Check sheet for the modelled part. Datum: model origin and axes. Units: mm. A direction names the side the tool comes from. Give positions to 0.01 mm unless a question says otherwise; leave off trailing zeros. Order: outer loops, then holes, each group sorted by start corner. A loop starts at its lowest first (then second) coordinate and runs counter-clockwise, first axis right, second up.
```python
from build123d import *

# Parameters (mm, degrees)
SKETCH1_R           = 1.5
BOSS_EXTRUDE1_DEPTH = 1
SKETCH2_R           = 1
BOSS_EXTRUDE2_DEPTH = 2.54


with BuildPart() as part:
    # Sketch1 → Boss-Extrude1 (new body, symmetric)
    with BuildSketch(Plane(origin=(0, 0, 0), x_dir=(1, 0, 0), z_dir=(0, 1, 0))):
        Circle(SKETCH1_R)
    extrude(amount=BOSS_EXTRUDE1_DEPTH, both=True)

    # Sketch2 → Boss-Extrude2 (add)
    with BuildSketch(Plane(origin=(0, 1, 0), x_dir=(1, 0, 0), z_dir=(0, 1, 0))):
        Circle(SKETCH2_R)
    boss_extrude2 = extrude(amount=BOSS_EXTRUDE2_DEPTH)

    # Mirror1: Boss-Extrude2 across plane
    add(boss_extrude2.mirror(Plane.ZX))


solid = part.part
```
(1) Set-up check for faces 1 (the face through (0, 2, 1)), 2 (the face through (0, -2, 1)), 3 (the face through (0, -3.54, 0)): record each of +Z, -Z, +X, -X, +Y, -Y from which the full face is reachable in a straight line by a thin tool's end or side.
Response values:
face 1: +Y
face 2: -Y
face 3: +Z, -Z, +X, -X, -Y
(2) Cross-section at B-B on z = 0. Enter the section's corners in (x, y), then the cut area to 3 significant figures.
Response values:
outline: (-1.5, -1) - (-1, -1) - (-1, -3.54) - (1, -3.54) - (1, -1) - (1.5, -1) - (1.5, 1) - (1, 1) - (1, 3.54) - (-1, 3.54) - (-1, 1) - (-1.5, 1) - close
area: 16.2 mm2
(3) Material ranges on L1, parallel to Y at x = -1, z = -0.85; L2, parallel to Z at x = 0.7, y = 1.5; L3, parallel to X at y = 1.25, z = -0.3, recorded low to high.
Response values:
L1: y = -1 to 1
L2: z = -0.71 to 0.71
L3: x = -0.95 to 0.95
(4) Cross-section at A-A on x = 0. Enter the section's corners in (y, z), then the cut area to 3 significant figures.
Response values:
outline: (-3.54, -1) - (-1, -1) - (-1, -1.5) - (1, -1.5) - (1, -1) - (3.54, -1) - (3.54, 1) - (1, 1) - (1, 1.5) - (-1, 1.5) - (-1, 1) - (-3.54, 1) - close
area: 16.2 mm2
(5) Cross-section at D-D on z = -1.2. Enter the section's corners in (x, y).
Response values:
outline: (-0.9, -1) - (0.9, -1) - (0.9, 1) - (-0.9, 1) - close
(6) Cross-section at C-C on y = -0.5. Enter the section's corners in (x, z), then the cut area to 3 significant figures.
Response values:
outline: circle Ø3 at (0, 0)
area: 7.07 mm2
